Here's how the part is built. I have some questions about the finished solid (model axes, mm). Face numbers are marked on the shaded views. A direction names the side the tool comes from. Round coordinates to 2 decimals unless told otherwise and drop trailing zeros. Order: outer loops, then holes, each group sorted by start corner. A loop starts at its lowest first (then second) coordinate and runs counter-clockwise, first axis right, second up. Notation, with made-up numbers: (-7.75, 47) -> (21.25, 47) arc R22 cw to (21.25, 64) -> close; hole circle Ø10 at (-37, -16). An arc over 180 degrees is marked (long way). Answer in a Markdown table with one row per item.
```python
from build123d import *

# Parameters (mm, degrees)
F0_R     = 13.97
F1_DEPTH = 15.24
F2_T     = -2.286
F3_R     = 0.508
F4_R     = 0.508


with BuildPart() as f1:
    # F0 (on Top) → F1 (new body)
    with BuildSketch(Plane.XY):
        Circle(F0_R)
    extrude(amount=F1_DEPTH)

    # F2
    f2_openings = [f1.faces().sort_by_distance(p)[0] for p in [
        (0, 0, 15.24),
    ]]
    offset(amount=F2_T, openings=f2_openings)

    # F3
    f3_edges = [f1.edges().sort_by_distance(p)[0] for p in [
        (-11.684, 0, 2.286),
    ]]
    fillet(f3_edges, radius=F3_R)

    # F4
    f4_edges = [f1.edges().sort_by_distance(p)[0] for p in [
        (-13.97, 0, 0),
    ]]
    fillet(f4_edges, radius=F4_R)


solid = f1.part
```
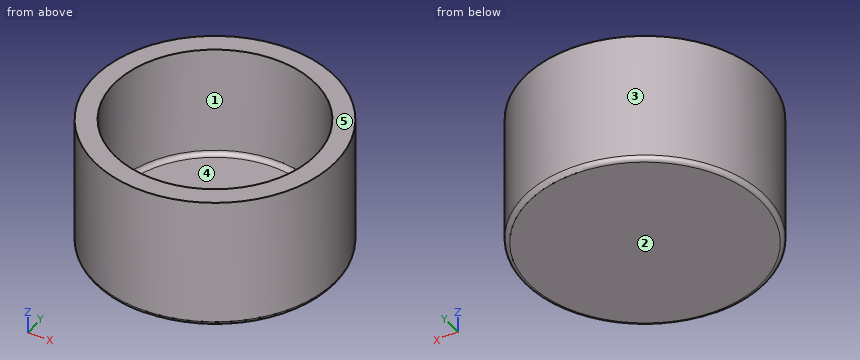
1. For the marked faces 1 and 2, which set-ups out of +Z, -Z, +X, -X, +Y, -Y let a thin tool reach every point of the face, with its end or its side?
Numbers:
| item | result |
|---|---|
| face 1 | +Z |
| face 2 | -Z, +X, -X, +Y, -Y |
2. For pin 1 Ø1 at (y, z) = (3.5, 11) entering from +X; pin 2 Ø6.5 at (x, y) = (5, -2) entering from +Z; pin 3 Ø1.5 at (x, z) = (-10, 3.5) entering from +Y, each with a flat end and sliding along its axis, tell me the tip position at first contact or that it passes through.
Numbers:
| item | result |
|---|---|
| pin 1 | stops at x = 13.64 |
| pin 2 | stops at z = 2.29 |
| pin 3 | stops at y = 10.47 |
3. We'd pull the mould along X, two halves only. Please class the marked faces 3, 4 and 5: released by +X, released by -X, zero draft, split by the parting line, or undercut.
Numbers:
| item | result |
|---|---|
| face 3 | split by the parting line |
| face 4 | undercut |
| face 5 | zero draft |
4. Please list where these lines run through material, in increasing order: line 1 along Y through (x, z) = (0, 6.25); line 2 along Z through (x, y) = (-8, -4.75); line 3 along X through (y, z) = (10, 4).
Numbers:
| item | result |
|---|---|
| line 1 | y = -13.97 to -11.68, 11.68 to 13.97 |
| line 2 | z = 0 to 2.29 |
| line 3 | x = -9.76 to -6.04, 6.04 to 9.76 |
5. Suppose I cut it at A-A on x = 0. Write out the boundary of the cut face in (y, z), then the cut area to 3 significant figures.
Numbers:
| item | result |
|---|---|
| outline | (-13.97, 0.51) arc R0.51 ccw to (-13.46, 0) -> (13.46, 0) arc R0.51 ccw to (13.97, 0.51) -> (13.97, 15.24) -> (11.68, 15.24) -> (11.68, 2.79) arc R0.51 cw to (11.18, 2.29) -> (-11.18, 2.29) arc R0.51 cw to (-11.68, 2.79) -> (-11.68, 15.24) -> (-13.97, 15.24) -> close |
| area | 123 mm2 |
6. Suppose I cut it at C-C on z = 6.5. Write out the boundary of the cut face in (x, y), then the cut area to 3 significant figures.
Numbers:
| item | result |
|---|---|
| outline | circle Ø27.94 at (0, 0); hole circle Ø23.37 at (0, 0) |
| area | 184 mm2 |
